Could you check a few things on this drawing? It's one solid part, dimensions in mm from its lowest x, y, z. A direction names the side the tool comes from. Coordinates: 2 decimals unless noted, no trailing zeros. Loops run counter-clockwise (first coordinate to the right, second up) from the corner with the lowest first, then second, coordinate; pieces in that order, holes last. Notation, with made-up numbers: (15, 1.5) -> (59, 1.5) arc R12 cw to (59, 10.5) -> close; hole circle Ø4 at (57, -21). An arc over 180 degrees is marked (long way). One line per question, with ' | ' between items. Start each with the question number.
(1) Suppose I cut it at D-D (z = 13). Please give me the cut outline in (x, y).
(2) If I drill on line 1 along X through (y, z) = (1.2, 13); line 2 along Y through (x, z) = (4.25, 6.5); line 3 along Z through (x, y) = (8, 1.2) (1 decimal), over which ranges is the centre line in solid material (lowest first)?
(3) I'm going to push a flat-ended pin straight in: pin 1 Ø0.6 at (y, z) = (1.5, 17.5) entering from -X. Where does the tip first touch, or does it pass through?
(4) Which directions (+Z, -Z, +X, -X, +Y, -Y) give clear straight access to the entire face, cutting with the end or side of a thin tool? Please do the marked faces 1 and 2.
(5) Suppose I cut it at C-C (y = 0.45). Please give me the cut outline in (x, z), plus the area to 3 significant figures.
(6) Suppose I cut it at B-B (z = 25.5). Please give me the cut outline in (x, y).
(7) Suppose I cut it at A-A (x = 17.5). Please give me the cut outline in (y, z).
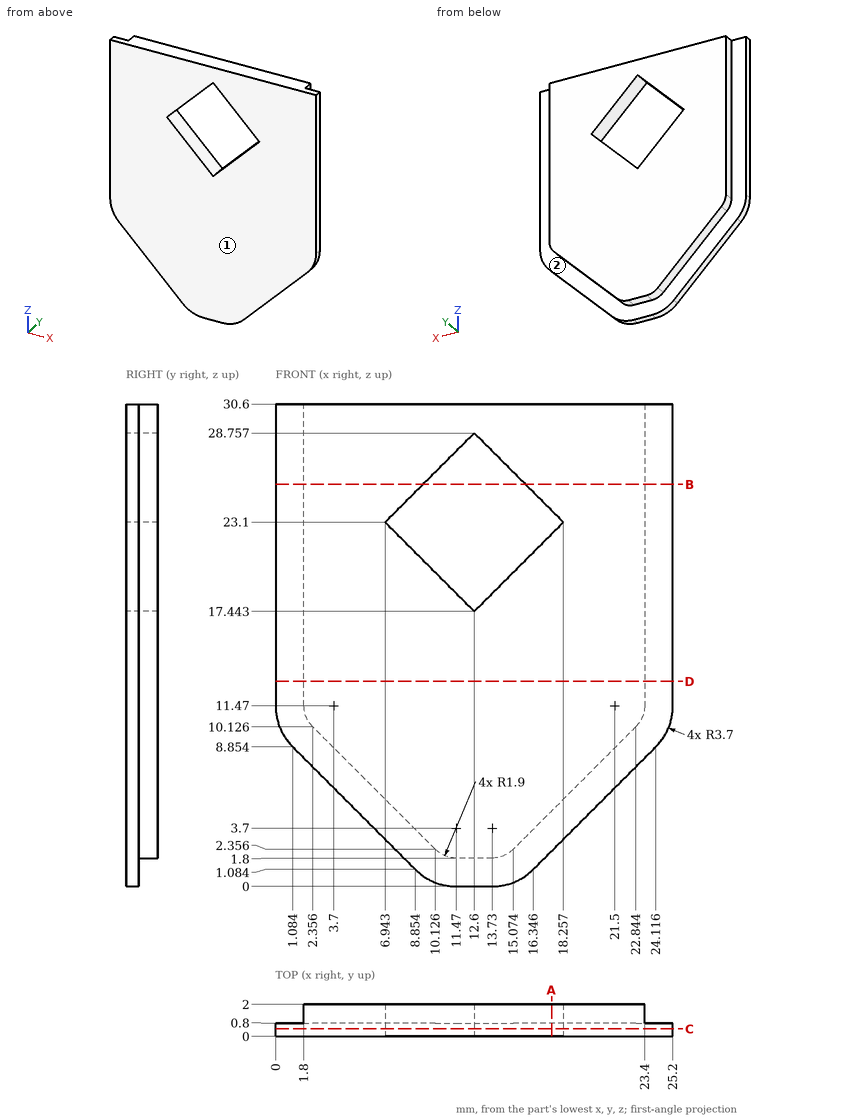
Checks:
1) outline: (0, 0) -> (25.2, 0) -> (25.2, 0.8) -> (23.4, 0.8) -> (23.4, 2) -> (1.8, 2) -> (1.8, 0.8) -> (0, 0.8) -> close
2) line 1: x = 1.8 to 23.4 | line 2: y = 0 to 0.8 | line 3: z = 4.5 to 22, 24.2 to 30.6
3) pin 1: stops at x = 1.8
4) face 1: +Z, -Z, +X, -X, -Y | face 2: -Z, +Y
5) outline: (0, 11.47) arc R3.7 ccw to (1.08, 8.85) -> (8.85, 1.08) arc R3.7 ccw to (11.47, 0) -> (13.73, 0) arc R3.7 ccw to (16.35, 1.08) -> (24.12, 8.85) arc R3.7 ccw to (25.2, 11.47) -> (25.2, 30.6) -> (0, 30.6) -> close; hole (6.94, 23.1) -> (12.6, 17.44) -> (18.26, 23.1) -> (12.6, 28.76) -> close | area: 607 mm^2
6) outline: (0, 0) -> (9.34, 0) -> (9.34, 2) -> (1.8, 2) -> (1.8, 0.8) -> (0, 0.8) -> close; (15.86, 0) -> (25.2, 0) -> (25.2, 0.8) -> (23.4, 0.8) -> (23.4, 2) -> (15.86, 2) -> close
7) outline: (0, 2.24) -> (0.8, 2.24) -> (0.8, 4.78) -> (2, 4.78) -> (2, 22.34) -> (0, 22.34) -> close; (0, 23.86) -> (2, 23.86) -> (2, 30.6) -> (0, 30.6) -> close
